The listing builds one solid part. Answer for the finished solid, in the listing's coordinates (mm). A direction names the side the tool comes from. Coordinates: 2 decimals unless noted, no trailing zeros. Loops run counter-clockwise (first coordinate to the right, second up) from the corner with the lowest first, then second, coordinate; pieces in that order, holes last. Notation, with made-up numbers: (87.5, -32.75) -> (129.5, -32.75) arc R16 cw to (129.5, -12.75) -> close; hole circle Ø11 at (-31, -25). An arc over 180 degrees is marked (long way). Answer in a Markdown table with one row per item.
```python
from build123d import *

# Parameters (mm, degrees)
SKETCH1_R           = 9.525
BOSS_EXTRUDE1_DEPTH = 6.35
EXTRUDE_THIN1_DEPTH = 88.9
SKETCH3_R           = 7.112
CUT_EXTRUDE1_DEPTH  = 77.2
CIRPATTERN1_COUNT   = 4


with BuildPart() as part:
    # Sketch1 → Boss-Extrude1 (new body)
    with BuildSketch(Plane.XY):
        with BuildLine():
            Line((-47.625, 76.2), (47.625, 76.2))
            ThreePointArc((47.625, 76.2), (49.87006403, 75.27006403), (50.8, 73.025))
            Line((50.8, 73.025), (50.8, -73.025))
            ThreePointArc((50.8, -73.025), (49.87006403, -75.27006403), (47.625, -76.2))
            Line((47.625, -76.2), (-47.625, -76.2))
            ThreePointArc((-47.625, -76.2), (-49.87006403, -75.27006403), (-50.8, -73.025))
            Line((-50.8, -73.025), (-50.8, 73.025))
            ThreePointArc((-50.8, 73.025), (-49.87006403, 75.27006403), (-47.625, 76.2))
        make_face()
        with Locations((0, 50.8)):
            Circle(SKETCH1_R, mode=Mode.SUBTRACT)
        with Locations((0, -50.8)):
            Circle(SKETCH1_R, mode=Mode.SUBTRACT)
    extrude(amount=BOSS_EXTRUDE1_DEPTH)

    # Sketch2 → Extrude-Thin1 (add)
    with BuildSketch(Plane.XY.offset(6.35)):
        with BuildLine():
            Line((-20.6375, 18.0975), (-20.6375, -18.0975))
            ThreePointArc((-20.6375, -18.0975), (-19.893551224, -19.893551224), (-18.0975, -20.6375))
            Line((-18.0975, -20.6375), (18.0975, -20.6375))
            ThreePointArc((18.0975, -20.6375), (19.893551224, -19.893551224), (20.6375, -18.0975))
            Line((20.6375, -18.0975), (20.6375, 18.0975))
            Line((20.6375, 18.0975), (26.9875, 18.0975))
            Line((26.9875, 18.0975), (26.9875, -18.0975))
            ThreePointArc((26.9875, -18.0975), (24.383679285, -24.383679285), (18.0975, -26.9875))
            Line((18.0975, -26.9875), (-18.0975, -26.9875))
            ThreePointArc((-18.0975, -26.9875), (-24.383679285, -24.383679285), (-26.9875, -18.0975))
            Line((-26.9875, -18.0975), (-26.9875, 18.0975))
            Line((-26.9875, 18.0975), (-20.6375, 18.0975))
        make_face()
    extrude(amount=EXTRUDE_THIN1_DEPTH)

    # Sketch3 → Cut-Extrude1 (cut, through all)
    with BuildSketch(Plane.XZ):
        with Locations((0, 74.6125)):
            Circle(SKETCH3_R)
        with Locations((0, 26.9875)):
            Circle(SKETCH3_R)
    cut_extrude1 = extrude(amount=CUT_EXTRUDE1_DEPTH, mode=Mode.SUBTRACT)

    # CirPattern1: Cut-Extrude1 ×4 about axis, 1 skipped
    cirpattern1_axis = Axis((0, 0, 74.6125), (0, 0, -1))
    add([cut_extrude1.rotate(cirpattern1_axis, i * 360 / CIRPATTERN1_COUNT) for i in range(1, CIRPATTERN1_COUNT) if i not in (2,)], mode=Mode.SUBTRACT)


solid = part.part
```
Item 1: Find the intervals of material crossed by probe 1 along X at (y, z) = (13.5, 38); probe 2 along Z at (x, y) = (-22.25, 0); probe 3 along Y at (x, z) = (0, 5) (3 decimals), in increasing order.
Findings below:
| item | result |
|---|---|
| probe 1 | x = -26.99 to -20.64, 20.64 to 26.99 |
| probe 2 | z = 0 to 19.88, 34.1 to 67.5, 81.72 to 95.25 |
| probe 3 | y = -76.2 to -60.325, -41.275 to 41.275, 60.325 to 76.2 |
Item 2: A cutting plane is placed at A-A, the plane y = 0. Determine the outline of the cut face in (x, z), plus the area to 3 significant figures.
Findings below:
| item | result |
|---|---|
| outline | (-50.8, 0) -> (50.8, 0) -> (50.8, 6.35) -> (26.99, 6.35) -> (26.99, 19.88) -> (20.64, 19.88) -> (20.64, 6.35) -> (-20.64, 6.35) -> (-20.64, 19.88) -> (-26.99, 19.88) -> (-26.99, 6.35) -> (-50.8, 6.35) -> close; (-26.99, 34.1) -> (-20.64, 34.1) -> (-20.64, 67.5) -> (-26.99, 67.5) -> close; (-26.99, 81.72) -> (-20.64, 81.72) -> (-20.64, 95.25) -> (-26.99, 95.25) -> close; (20.64, 34.1) -> (26.99, 34.1) -> (26.99, 67.5) -> (20.64, 67.5) -> close; (20.64, 81.72) -> (26.99, 81.72) -> (26.99, 95.25) -> (20.64, 95.25) -> close |
| area | 1,410 mm2 |
Item 3: A cutting plane is placed at C-C, the plane y = 50.8. Determine the outline of the cut face in (x, z) (3 decimals).
Findings below:
| item | result |
|---|---|
| outline | (-50.8, 0) -> (-9.525, 0) -> (-9.525, 6.35) -> (-50.8, 6.35) -> close; (9.525, 0) -> (50.8, 0) -> (50.8, 6.35) -> (9.525, 6.35) -> close |
Item 4: A cutting plane is placed at B-B, the plane x = 0. Count the separate pieces of the cut face and the enclosed holes in it, plus the area to 3 significant figures.
Findings below:
| item | result |
|---|---|
| separate pieces | 5 |
| enclosed holes | 0 |
| area | 1,110 mm2 |
Item 5: Flat-ended cylindrical pins translate along their axes: pin 1 Ø1 at (x, y) = (-14, 55.5) entering from -Z; pin 2 Ø1.9 at (x, z) = (24.5, 55) entering from +Y; pin 3 Ø11 at (x, z) = (-6.5, 52.5) entering from -Y; pin 4 Ø16.5 at (x, z) = (0, 74.61) entering from +Y. Find the tip coordinate at first contact, or state that the pin passes through.
Findings below:
| item | result |
|---|---|
| pin 1 | stops at z = 0 |
| pin 2 | stops at y = 18.1 |
| pin 3 | stops at y = -26.99 |
| pin 4 | stops at y = -20.64 |
Item 6: A cutting plane is placed at D-D, the plane z = 71.5. Determine the outline of the cut face in (x, y), plus the area to 3 significant figures.
Findings below:
| item | result |
|---|---|
| outline | (-26.99, -18.1) arc R8.89 ccw to (-18.1, -26.99) -> (-6.39, -26.99) -> (-6.39, -20.64) -> (-18.1, -20.64) arc R2.54 cw to (-20.64, -18.1) -> (-20.64, -6.39) -> (-26.99, -6.39) -> close; (-26.99, 6.39) -> (-20.64, 6.39) -> (-20.64, 18.1) -> (-26.99, 18.1) -> close; (6.39, -26.99) -> (18.1, -26.99) arc R8.89 ccw to (26.99, -18.1) -> (26.99, -6.39) -> (20.64, -6.39) -> (20.64, -18.1) arc R2.54 cw to (18.1, -20.64) -> (6.39, -20.64) -> close; (20.64, 6.39) -> (26.99, 6.39) -> (26.99, 18.1) -> (20.64, 18.1) -> close |
| area | 560 mm2 |
Item 7: Determine the mould class of faces 4 (the face through (-23.77, 0.93, 34.04)), 5 (the face through (1, 1, 6.35)), 6 (the face through (1, 1, 0)) for opening direction Z: +Z half, -Z half, draft (parallel to the pull), parting line (faces both ways), or undercut.
Findings below:
| item | result |
|---|---|
| face 4 | undercut |
| face 5 | +Z half |
| face 6 | -Z half |
Item 8: A tool of negligible diameter and unlimited length cuts with its end or side. For faces 1 (the face through (26.988, 0, 50)), 2 (the face through (-24, 18.098, 50)), 3 (the face through (0, -20.638, 50)), from which of +Z, -Z, +X, -X, +Y, -Y can it reach the whole face along a straight path? Write none if from no direction.
Findings below:
| item | result |
|---|---|
| face 1 | +Z, +X, +Y, -Y |
| face 2 | +Z, +X, -X, +Y |
| face 3 | +Z, +Y |
